Read the model definition and answer for the solid it produces. Units are mm, in the model's axes. A direction names the side the tool comes from. Round coordinates to 2 decimals unless told otherwise and drop trailing zeros. Order: outer loops, then holes, each group sorted by start corner. A loop starts at its lowest first (then second) coordinate and runs counter-clockwise, first axis right, second up.
from build123d import *

# Parameters (mm, degrees)
SKETCH1_W                                         = 50.8
SKETCH1_H                                         = 50.8
BOSS_EXTRUDE1_DEPTH                               = 6.35
CUT_EXTRUDE1_DEPTH                                = 7.35
CUT_EXTRUDE2_DASH_027_DEPTH                       = 1.3208
CSK_FOR_6_FLAT_HEAD_MACHINE_SCREW_100_D           = 3.7973
CSK_FOR_6_FLAT_HEAD_MACHINE_SCREW_100_CSINK_D     = 7.0866
CSK_FOR_6_FLAT_HEAD_MACHINE_SCREW_100_CSINK_ANGLE = 100
CSK_FOR_4_FLAT_HEAD_MACHINE_SCREW_100_D           = 3.2639
CSK_FOR_4_FLAT_HEAD_MACHINE_SCREW_100_CSINK_D     = 6.477
CSK_FOR_4_FLAT_HEAD_MACHINE_SCREW_100_CSINK_ANGLE = 82
SKETCH8_R                                         = 4.826
CUT_EXTRUDE2_DEPTH                                = 7.35


with BuildPart() as part:
    # Sketch1 → Boss-Extrude1 (new body)
    with BuildSketch(Plane.XY):
        Rectangle(SKETCH1_W, SKETCH1_H)
    extrude(amount=BOSS_EXTRUDE1_DEPTH)

    # Sketch2 → Cut-Extrude1 (cut, through all)
    with BuildSketch(Plane.XY.offset(6.35)):
        with BuildLine():
            Line((-4.7625, -15.875), (4.7625, -15.875))
            ThreePointArc((4.7625, -15.875), (8.130096045, -14.480096045), (9.525, -11.1125))
            Line((9.525, -11.1125), (9.525, 11.1125))
            ThreePointArc((9.525, 11.1125), (8.130096045, 14.480096045), (4.7625, 15.875))
            Line((4.7625, 15.875), (-4.7625, 15.875))
            ThreePointArc((-4.7625, 15.875), (-8.130096045, 14.480096045), (-9.525, 11.1125))
            Line((-9.525, 11.1125), (-9.525, -11.1125))
            ThreePointArc((-9.525, -11.1125), (-8.130096045, -14.480096045), (-4.7625, -15.875))
        make_face()
    extrude(amount=-CUT_EXTRUDE1_DEPTH, mode=Mode.SUBTRACT)

    # Sketch3 → Cut-Extrude2 - dash 027 (cut)
    with BuildSketch(Plane.XY.offset(6.35)):
        with BuildLine():
            Line((13.3477, -11.176), (13.3477, 11.176))
            ThreePointArc((13.3477, 11.176), (10.848032113, 17.210732113), (4.8133, 19.7104))
            Line((4.8133, 19.7104), (-4.8133, 19.7104))
            ThreePointArc((-4.8133, 19.7104), (-10.848032113, 17.210732113), (-13.3477, 11.176))
            Line((-13.3477, 11.176), (-13.3477, -11.176))
            ThreePointArc((-13.3477, -11.176), (-10.848032113, -17.210732113), (-4.8133, -19.7104))
            Line((-4.8133, -19.7104), (4.8133, -19.7104))
            ThreePointArc((4.8133, -19.7104), (10.848032113, -17.210732113), (13.3477, -11.176))
        make_face()
        with BuildLine():
            Line((-4.8133, -17.526), (4.8133, -17.526))
            ThreePointArc((4.8133, -17.526), (9.303428061, -15.666128061), (11.1633, -11.176))
            Line((11.1633, -11.176), (11.1633, 11.176))
            ThreePointArc((11.1633, 11.176), (9.303428061, 15.666128061), (4.8133, 17.526))
            Line((4.8133, 17.526), (-4.8133, 17.526))
            ThreePointArc((-4.8133, 17.526), (-9.303428061, 15.666128061), (-11.1633, 11.176))
            Line((-11.1633, 11.176), (-11.1633, -11.176))
            ThreePointArc((-11.1633, -11.176), (-9.303428061, -15.666128061), (-4.8133, -17.526))
        make_face(mode=Mode.SUBTRACT)
    cut_extrude2_dash_027 = extrude(amount=-CUT_EXTRUDE2_DASH_027_DEPTH, mode=Mode.SUBTRACT)

    # CSK for #6 Flat Head Machine Screw (100)1 (through all)
    with Locations(Plane.XY.offset(6.35)):
        with Locations((-20.6375, 20.6375), (20.6375, 20.6375), (20.6375, -20.6375), (-20.6375, -20.6375)):
            CounterSinkHole(CSK_FOR_6_FLAT_HEAD_MACHINE_SCREW_100_D / 2, CSK_FOR_6_FLAT_HEAD_MACHINE_SCREW_100_CSINK_D / 2, counter_sink_angle=CSK_FOR_6_FLAT_HEAD_MACHINE_SCREW_100_CSINK_ANGLE)

    # CSK for #4 Flat Head Machine Screw (100)1 (through all)
    with Locations(Plane(origin=(0, 0, 0), x_dir=(-1, 0, 0), z_dir=(0, 0, -1))):
        with Locations((-11.90625, 21.43125), (11.90625, 21.43125), (-11.90625, -21.43125), (11.90625, -21.43125)):
            CounterSinkHole(CSK_FOR_4_FLAT_HEAD_MACHINE_SCREW_100_D / 2, CSK_FOR_4_FLAT_HEAD_MACHINE_SCREW_100_CSINK_D / 2, counter_sink_angle=CSK_FOR_4_FLAT_HEAD_MACHINE_SCREW_100_CSINK_ANGLE)

    # Mirror1: Cut-Extrude2 - dash 027 across plane
    add(cut_extrude2_dash_027.mirror(Plane(origin=(0, 0, 3.175), x_dir=(1, 0, 0), z_dir=(0, 0, -1))), mode=Mode.SUBTRACT)

    # Sketch8 → Cut-Extrude2 (cut, through all)
    with BuildSketch(Plane.XY.offset(6.35)):
        with Locations((-25.6921, 5.334)):
            Circle(SKETCH8_R)
    cut_extrude2 = extrude(amount=-CUT_EXTRUDE2_DEPTH, mode=Mode.SUBTRACT)

    # Mirror2: Cut-Extrude2 across plane
    add(cut_extrude2.mirror(Plane(origin=(0, 0, 0), x_dir=(0, 0, 1), z_dir=(1, 0, 0))), mode=Mode.SUBTRACT)


solid = part.part
Q1. For a pull along Y with two mould halves and no side action, classify faces 4 (the face through (-9.35, -15.62, 0.65)), 5 (the face through (-10.78, 17.28, 0.65)), 6 (the face through (-25.4, 18, 3)) as released by +Y, released by -Y, zero draft, split by the parting line, or undercut.
Outcome:
face 4: undercut
face 5: undercut
face 6: zero draft
Q2. A cutting plane is placed at A-A, the plane y = -2. Give the vertices of the cut face in (x, z) (3 decimals), plus the area to 3 significant figures.
Outcome:
outline: (-25.4, 0) - (-13.348, 0) - (-13.348, 1.321) - (-11.163, 1.321) - (-11.163, 0) - (-9.525, 0) - (-9.525, 6.35) - (-11.163, 6.35) - (-11.163, 5.029) - (-13.348, 5.029) - (-13.348, 6.35) - (-25.4, 6.35) - close; (9.525, 0) - (11.163, 0) - (11.163, 1.321) - (13.348, 1.321) - (13.348, 0) - (25.4, 0) - (25.4, 6.35) - (13.348, 6.35) - (13.348, 5.029) - (11.163, 5.029) - (11.163, 6.35) - (9.525, 6.35) - close
area: 190 mm2
Q3. Straight lines are drawn through the part: probe 1 along Y at (x, z) = (-1.5, 2.5) (3 decimals); probe 2 along Y at (x, z) = (-20.5, 3.5); probe 3 along X at (y, z) = (9, 0.5) (3 decimals). For each, find the intervals that lie inside material, in ascending order.
Outcome:
probe 1: y = -25.4 to -15.875, 15.875 to 25.4
probe 2: y = -25.4 to -22.53, -18.74 to 18.74, 22.53 to 25.4
probe 3: x = -22.554 to -13.348, -11.163 to -9.525, 9.525 to 11.163, 13.348 to 22.554
Q4. For faces 1 (the face through (0, -15.875, 3)), 2 (the face through (-11.163, 0, 1)), 3 (the face through (9.35, 15.62, 5.7)), determine the directions among +Z, -Z, +X, -X, +Y, -Y from which every point of the face is accessible in a straight line to the end or side of a thin tool.
Outcome:
face 1: +Z, -Z
face 2: -Z
face 3: +Z
Q5. A flat-ended cylindrical pin translates along its axis: pin 1 (6 mm diameter, centred on x = 20.64, y = 20.64, fed in from +Z). Find the tip coordinate at first contact, or state that the pin passes through.
Outcome:
pin 1: stops at z = 5.9
Q6. A cutting plane is placed at D-D, the plane y = -16.5. Give the vertices of the cut face in (x, z), plus the area to 3 significant figures.
Outcome:
outline: (-25.4, 0) - (-11.48, 0) - (-11.48, 1.32) - (-8.27, 1.32) - (-8.27, 0) - (8.27, 0) - (8.27, 1.32) - (11.48, 1.32) - (11.48, 0) - (25.4, 0) - (25.4, 6.35) - (11.48, 6.35) - (11.48, 5.03) - (8.27, 5.03) - (8.27, 6.35) - (-8.27, 6.35) - (-8.27, 5.03) - (-11.48, 5.03) - (-11.48, 6.35) - (-25.4, 6.35) - close
area: 306 mm2
Q7. A cutting plane is placed at B-B, the plane x = -1. Give the vertices of the cut face in (y, z) (3 decimals), plus the area to 3 significant figures.
Outcome:
outline: (-25.4, 0) - (-19.71, 0) - (-19.71, 1.321) - (-17.526, 1.321) - (-17.526, 0) - (-15.875, 0) - (-15.875, 6.35) - (-17.526, 6.35) - (-17.526, 5.029) - (-19.71, 5.029) - (-19.71, 6.35) - (-25.4, 6.35) - close; (15.875, 0) - (17.526, 0) - (17.526, 1.321) - (19.71, 1.321) - (19.71, 0) - (25.4, 0) - (25.4, 6.35) - (19.71, 6.35) - (19.71, 5.029) - (17.526, 5.029) - (17.526, 6.35) - (15.875, 6.35) - close
area: 109 mm2
Q8. A cutting plane is placed at C-C, the plane z = 2.5. Give the number of separate pieces and of enclosed holes in the cut face, plus the area to 3 significant figures.
Outcome:
separate pieces: 1
enclosed holes: 9
area: 1,850 mm2
